Here's how the part is built. I have some questions about the finished solid (model axes, mm). Round coordinates to 2 decimals unless told otherwise and drop trailing zeros. Write each loop counter-clockwise with the first axis right and the second up, starting at its lowest first coordinate (ties: lowest second). Pieces come first, ordered by that corner, then holes. Notation, with made-up numbers: (-8, 38.5) - (31, 38.5) arc R11 cw to (31, 57.5) - close; hole circle Ø11 at (-28.5, 21.5). An arc over 180 degrees is marked (long way). Return JSON: item names as keys, results as strings. Group by question number.
```python
from build123d import *

# Parameters (mm, degrees)
SKETCH2_W           = 84
SKETCH2_H           = 24
SKETCH2_W_2         = 70
SKETCH2_H_2         = 10
BOSS_EXTRUDE1_DEPTH = 4
SKETCH3_W           = 77
SKETCH3_H           = 17
SKETCH3_W_2         = 70
SKETCH3_H_2         = 10
BOSS_EXTRUDE2_DEPTH = 9
DRAFT2_ANGLE        = 4
FILLET2_R           = 4
FILLET1_R           = 1
FILLET3_R           = 1


with BuildPart() as part:
    # Sketch2 → Boss-Extrude1 (new body)
    with BuildSketch(Plane.XY):
        Rectangle(SKETCH2_W, SKETCH2_H)
        Rectangle(SKETCH2_W_2, SKETCH2_H_2, mode=Mode.SUBTRACT)
    extrude(amount=BOSS_EXTRUDE1_DEPTH)

    # Sketch3 → Boss-Extrude2 (add)
    with BuildSketch(Plane.XY):
        Rectangle(SKETCH3_W, SKETCH3_H)
        Rectangle(SKETCH3_W_2, SKETCH3_H_2, mode=Mode.SUBTRACT)
    extrude(amount=-BOSS_EXTRUDE2_DEPTH)

    # Draft2
    draft2_faces = [part.faces().sort_by_distance(p)[0] for p in [
        (0, 8.5, -4.5),
        (-38.5, 0, -4.5),
        (38.5, 0, -4.5),
        (0, -8.5, -4.5),
    ]]
    draft(draft2_faces, Plane(origin=(0, 0, 0), x_dir=(-1, 0, 0), z_dir=(0, 0, -1)), DRAFT2_ANGLE)

    # Fillet2
    fillet2_edges = [part.edges().sort_by_distance(p)[0] for p in [
        (35, -5, -2.5),
        (35, 5, -2.5),
        (-35, 5, -2.5),
        (-35, -5, -2.5),
        (42, -12, 2),
        (-42, -12, 2),
        (-42, 12, 2),
        (42, 12, 2),
    ]]
    fillet(fillet2_edges, radius=FILLET2_R)

    # Fillet1
    fillet1_edges = [part.edges().sort_by_distance(p)[0] for p in [
        (0, -12, 4),
        (-42, 0, 4),
        (42, 0, 4),
        (0, 12, 4),
        (0, 5, 4),
        (35, 0, 4),
        (0, -5, 4),
        (-35, 0, 4),
        (40.828427125, -10.828427125, 4),
        (40.828427125, 10.828427125, 4),
        (-40.828427125, 10.828427125, 4),
        (-40.828427125, -10.828427125, 4),
        (33.828427125, 3.828427125, 4),
        (-33.828427125, 3.828427125, 4),
        (-33.828427125, -3.828427125, 4),
        (33.828427125, -3.828427125, 4),
    ]]
    fillet(fillet1_edges, radius=FILLET1_R)

    # Fillet3
    fillet3_edges = [part.edges().sort_by_distance(p)[0] for p in [
        (-38.185329346, -8.185329346, -4.5),
        (-38.185329346, 8.185329346, -4.5),
        (38.185329346, 8.185329346, -4.5),
        (38.185329346, -8.185329346, -4.5),
    ]]
    fillet(fillet3_edges, radius=FILLET3_R)


solid = part.part
```
1) Imagine slicing it at A-A (x = 26). Please give me the cut outline in (y, z).
2) I need wall thicknesses on line 1 along Y through (x, z) = (-1, -7); line 2 along Y through (x, z) = (-12, 2.5); line 3 along Z through (x, y) = (-2, -10.25). Which ranges of each line are inside material? Lowest first, please.
3) Will these pins go through, and if not, where does the flat tip stop? pin 1 Ø6 at (x, z) = (9, -5) entering from +Y; pin 2 Ø5 at (x, y) = (-14.5, -1) entering from +Z; pin 3 Ø1 at (x, z) = (28.5, -4) entering from +Y; pin 4 Ø3 at (x, z) = (10.5, -7.5) entering from -Y.
4) If we mould it in two halves opening along Y, with no side actions, what happens to faces 1 (the cylindrical face through (-33.859, -3.797, -2.916)), 2 (the cylindrical face through (-33.859, 3.797, -3.084)), 3 (the cylindrical face through (40.859, 10.797, 1.521)), 4 (the flat face through (-1, -12, 1))? For each: released by +Y, released by -Y, zero draft, split by the parting line, or undercut.
Results found:
{
 "1": {"outline": "(-12, 0) - (-8.5, 0) - (-7.87, -9) - (-5, -9) - (-5, 3) arc R1 ccw to (-6, 4) - (-11, 4) arc R1 ccw to (-12, 3) - close; (5, -9) - (7.87, -9) - (8.5, 0) - (12, 0) - (12, 3) arc R1 ccw to (11, 4) - (6, 4) arc R1 ccw to (5, 3) - close"},
 "2": {"line 1": "y = -8.01 to -5, 5 to 8.01", "line 2": "y = -12 to -5, 5 to 12", "line 3": "z = 0 to 4"},
 "3": {"pin 1": "stops at y = 8.36", "pin 2": "passes through", "pin 3": "stops at y = 8.26", "pin 4": "stops at y = -8.08"},
 "4": {"face 1": "undercut", "face 2": "undercut", "face 3": "released by +Y", "face 4": "released by -Y"}
}
